Could you check a few things on this model? Use its own coordinates, in mm. A direction names the side the tool comes from. Coordinates: 2 decimals unless noted, no trailing zeros. Order: outer loops, then holes, each group sorted by start corner. A loop starts at its lowest first (then second) coordinate and runs counter-clockwise, first axis right, second up. Notation, with made-up numbers: (56, 36.5) -> (99, 36.5) arc R19 ccw to (99, 64.5) -> close; hole circle Ø8 at (77, 12.5). An arc over 180 degrees is marked (long way). Use a Markdown table: item, result. Add a question column.
1) If I drill on L1, parallel to X at y = 5, z = 0.7; L2, parallel to Y at x = 15, z = 0.3, over which ranges is the centre line in solid material (lowest first)? Write a range as [from, to].
2) If we section it at A-A (x = 15): Write out the boundary of the cut face in (y, z), plus the area to 3 significant figures.
3) If we section it at C-C (z = 0.6): Write out the boundary of the cut face in (x, y), plus the area to 3 significant figures.
4) Which directions (+Z, -Z, +X, -X, +Y, -Y) give clear straight access to the entire face, cutting with the end or side of a thin tool? Please do faces 4 (the flat face through (19, 25.4, 0.5)), 5 (the flat face through (4.4, 19, 0.5)), 6 (the flat face through (14.9, 9, 0.5)).
5) Will this pin go through, and if not, where does the flat tip stop? pin 1 Ø6 at (x, y) = (15, 15) entering from +Z.
6) Thinking about a two-plate mould opening in X: for faces 1 (the flat face through (30, 24.4, 0.5)), 2 (the flat face through (11, 25.4, 0.5)), 3 (the flat face through (24.4, 30, 0.5)), which applies, +X half, -X half, draft (parallel to the pull), parting line (faces both ways), or undercut?
```python
from build123d import *

# Parameters (mm, degrees)
SKETCH003_W   = 30
SKETCH003_H   = 30
PAD002_DEPTH  = 1
SKETCH002_R   = 3.65
SKETCH002_W   = 8
SKETCH002_H   = 9
SKETCH002_W_2 = 9
SKETCH002_H_2 = 8
POCKET_DEPTH  = 1


with BuildPart() as part:
    # Sketch003 → Pad002 (new body)
    with BuildSketch(Plane.XY):
        with Locations((15, 15)):
            Rectangle(SKETCH003_W, SKETCH003_H)
    extrude(amount=PAD002_DEPTH)

    # Sketch002 → Pocket (cut)
    with BuildSketch(Plane.XY.offset(1)):
        with Locations((15, 15)):
            Circle(SKETCH002_R)
        with Locations((15, 25.5)):
            Rectangle(SKETCH002_W, SKETCH002_H)
        with Locations((15, 4.5)):
            Rectangle(SKETCH002_W, SKETCH002_H)
        with Locations((4.5, 15)):
            Rectangle(SKETCH002_W_2, SKETCH002_H_2)
        with Locations((25.5, 15)):
            Rectangle(SKETCH002_W_2, SKETCH002_H_2)
    extrude(amount=-POCKET_DEPTH, mode=Mode.SUBTRACT)


solid = part.part
```
Answer sheet:
| question | item | result |
|---|---|---|
| 1 | L1 | [0, 11], [19, 30] |
| 1 | L2 | [9, 11.35], [18.65, 21] |
| 2 | outline | (9, 0) -> (11.35, 0) -> (11.35, 1) -> (9, 1) -> close; (18.65, 0) -> (21, 0) -> (21, 1) -> (18.65, 1) -> close |
| 2 | area | 4.70 mm2 |
| 3 | outline | (0, 0) -> (11, 0) -> (11, 9) -> (19, 9) -> (19, 0) -> (30, 0) -> (30, 11) -> (21, 11) -> (21, 19) -> (30, 19) -> (30, 30) -> (19, 30) -> (19, 21) -> (11, 21) -> (11, 30) -> (0, 30) -> (0, 19) -> (9, 19) -> (9, 11) -> (0, 11) -> close; hole circle Ø7.3 at (15, 15) |
| 3 | area | 570 mm2 |
| 4 | face 4 | +Z, -Z, +Y |
| 4 | face 5 | +Z, -Z, -X |
| 4 | face 6 | +Z, -Z, -Y |
| 5 | pin 1 | through |
| 6 | face 1 | +X half |
| 6 | face 2 | undercut |
| 6 | face 3 | draft |
